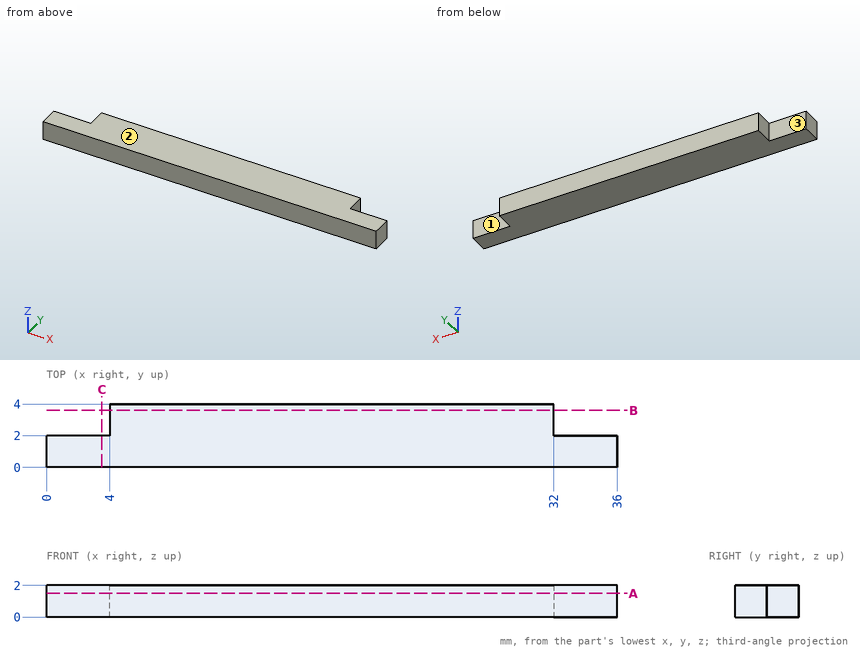
Verification items for this drawing (mm, ordinates from the low corner). A direction names the side the tool comes from. Round coordinates to 2 decimals unless told otherwise and drop trailing zeros. Loops run counter-clockwise (first coordinate to the right, second up) from the corner with the lowest first, then second, coordinate; pieces in that order, holes last. Notation, with made-up numbers: (63.25, 78.5) - (122.25, 78.5) arc R13 cw to (122.25, 88.5) - close; hole circle Ø7 at (14.25, 53.25). An arc over 180 degrees is marked (long way). Answer as CSV lines item,"result". Start each with the question number.
Item 1: Section check A-A (z = 1.5). Record the boundary of the cut face in (x, y), and give its area (3 significant figures).
Item 2: Set-up check for the marked faces 1, 2 and 3: record each of +Z, -Z, +X, -X, +Y, -Y from which the full face is reachable in a straight line by a thin tool's end or side.
Item 3: Section check B-B (y = 3.6). Record the boundary of the cut face in (x, z), and give its area (3 significant figures).
Item 4: Section check C-C (x = 3.5). Record the boundary of the cut face in (y, z), and give its area (3 significant figures).
Item 5: Depth check by flat-ended pin: P1, Ø1, axis at x = 2.5, z = 0.5, coming from the +Y side. Enter the tip coordinate at first touch or a pass-through.
Item 6: Scan lines: line 1 (X direction, y = 3, z = 0.2); line 2 (Y direction, x = 32.5, z = 0.55). Record each from-to range of solid material in increasing order. Write a range as [from, to].
Report:
1,outline,"(0, 0) - (36, 0) - (36, 2) - (32, 2) - (32, 4) - (4, 4) - (4, 2) - (0, 2) - close"
1,area,"128 mm2"
2,face 1,"+Z, -Z, +X, +Y"
2,face 2,"+Z, +X, -X, +Y, -Y"
2,face 3,"+Z, -Z, -X, +Y"
3,outline,"(4, 0) - (32, 0) - (32, 2) - (4, 2) - close"
3,area,"56.0 mm2"
4,outline,"(0, 0) - (2, 0) - (2, 2) - (0, 2) - close"
4,area,"4.00 mm2"
5,P1,"stops at y = 2"
6,line 1,"x = [4, 32]"
6,line 2,"y = [0, 2]"
